```python
from build123d import *

# Parameters (mm, degrees)
F1_DEPTH = 18
F2_R     = 8


with BuildPart() as f1:
    # F0 (on Front) → F1 (new body)
    with BuildSketch(Plane.XZ):
        with BuildLine():
            ThreePointArc((-57.712653, -188.988174), (-51.854789, -203.130309), (-37.712653, -208.988174))
            Line((-37.712653, -208.988174), (72.287347, -208.988174))
            ThreePointArc((72.287347, -208.988174), (86.429482, -203.130309), (92.287347, -188.988174))
            Line((92.287347, -188.988174), (92.287347, -48.988174))
            Line((92.287347, -48.988174), (92.287347, 44.301756))
            Line((92.287347, 44.301756), (92.287347, 91.011826))
            Line((92.287347, 91.011826), (-57.712653, 91.011826))
            Line((-57.712653, 91.011826), (-57.712653, -188.988174))
        make_face()
        with BuildLine():
            Line((92.287347, 44.301756), (92.287347, -48.988174))
            Line((92.287347, -48.988174), (116.240627, -48.988174))
            ThreePointArc((116.240627, -48.988174), (144.524898, -37.272445), (156.240627, -8.988174))
            Line((156.240627, -8.988174), (156.240627, 24.301756))
            ThreePointArc((156.240627, 24.301756), (150.382763, 38.443891), (136.240627, 44.301756))
            Line((136.240627, 44.301756), (92.287347, 44.301756))
        make_face()
    extrude(amount=F1_DEPTH)

    # F2
    f2_edges = [f1.edges().sort_by_distance(p)[0] for p in [
        (-57.712653, -18, -48.988174),
        (-57.712653, 0, -48.988174),
        (17.287347, -18, 91.011826),
        (17.287347, 0, 91.011826),
        (92.287347, -18, 67.656791),
        (92.287347, 0, 67.656791),
        (114.263987, 0, 44.301756),
        (114.263987, -18, 44.301756),
        (150.382763, 0, 38.443891),
    ]]
    fillet(f2_edges, radius=F2_R)


with BuildPart() as f1_1:
    # F3: moved
    add(f1.part.moved(Location((5, 0, 0))))


solid = f1_1.part
```
Part model, mm, in its own coordinate system. A direction names the side the tool comes from. Round coordinates to 2 decimals unless told otherwise and drop trailing zeros. Write each loop counter-clockwise with the first axis right and the second up, starting at its lowest first coordinate (ties: lowest second). Pieces come first, ordered by that corner, then holes.
Item 1: Probe L1, parallel to X at y = -7.75, z = -165.5; L2, parallel to Z at x = 106, y = -14; L3, parallel to X at y = -4.25, z = 60. List the from-to ranges inside material, lowest first.
Results:
L1: x = -52.71 to 97.28
L2: z = -47.92 to 43.23
L3: x = -51.78 to 96.35
Item 2: Drop flat-ended pins along their axis: pin 1 Ø1.5 at (x, y) = (19, -7) entering from +Z; pin 2 Ø2 at (y, z) = (-9, -145.5) entering from +X; pin 3 Ø1 at (x, y) = (106, -9) entering from -Z. Give the stop position or say it passes through.
Results:
pin 1: stops at z = 91.01
pin 2: stops at x = 97.29
pin 3: stops at z = -48.99
Item 3: Which spindle directions (+Z, -Z, +X, -X, +Y, -Y) get a long thin tool onto all of the face, cutting with end or side? Do faces 1 (the cylindrical face through (114.9, -2.406, 42.02)), 2 (the cylindrical face through (95, -2.4, -114)), 3 (the cylindrical face through (95, -15.6, -114)), 4 (the cylindrical face through (114.9, -15.594, 42.02)), 5 (the cylindrical face through (149.212, -8.986, -37.582)). Say none if no direction does.
Results:
face 1: +Z, +X, +Y
face 2: -Z, +X, +Y
face 3: -Z, +X, -Y
face 4: +Z, +X, -Y
face 5: -Z, +X, +Y, -Y
Item 4: Cut at B-B, the plane x = 106.5. Give the cut face in (y, z), plus the area to 3 significant figures.
Results:
outline: (-18, -40.99) arc R8 ccw to (-10, -48.99) - (-8, -48.99) arc R8 ccw to (0, -40.99) - (0, 36.3) arc R8 ccw to (-8, 44.3) - (-10, 44.3) arc R8 ccw to (-18, 36.3) - close
area: 1,620 mm2
Item 5: Cut at C-C, the plane y = -14.5. Give the cut face in (x, z) (3 decimals).
Results:
outline: (-51.327, -188.988) arc R18.614 ccw to (-32.713, -207.603) - (77.287, -207.603) arc R18.614 ccw to (95.902, -188.988) - (95.902, -47.603) - (121.241, -47.603) arc R38.614 ccw to (159.855, -8.988) - (159.855, 24.302) arc R18.614 ccw to (141.241, 42.916) - (95.902, 42.916) - (95.902, 89.626) - (-51.327, 89.626) - close
Item 6: Cut at A-A, the plane z = -112. Give the cut face in (x, y), plus the area to 3 significant figures.
Results:
outline: (-52.71, -10) arc R8 ccw to (-44.71, -18) - (89.29, -18) arc R8 ccw to (97.29, -10) - (97.29, -8) arc R8 ccw to (89.29, 0) - (-44.71, 0) arc R8 ccw to (-52.71, -8) - close
area: 2,650 mm2
